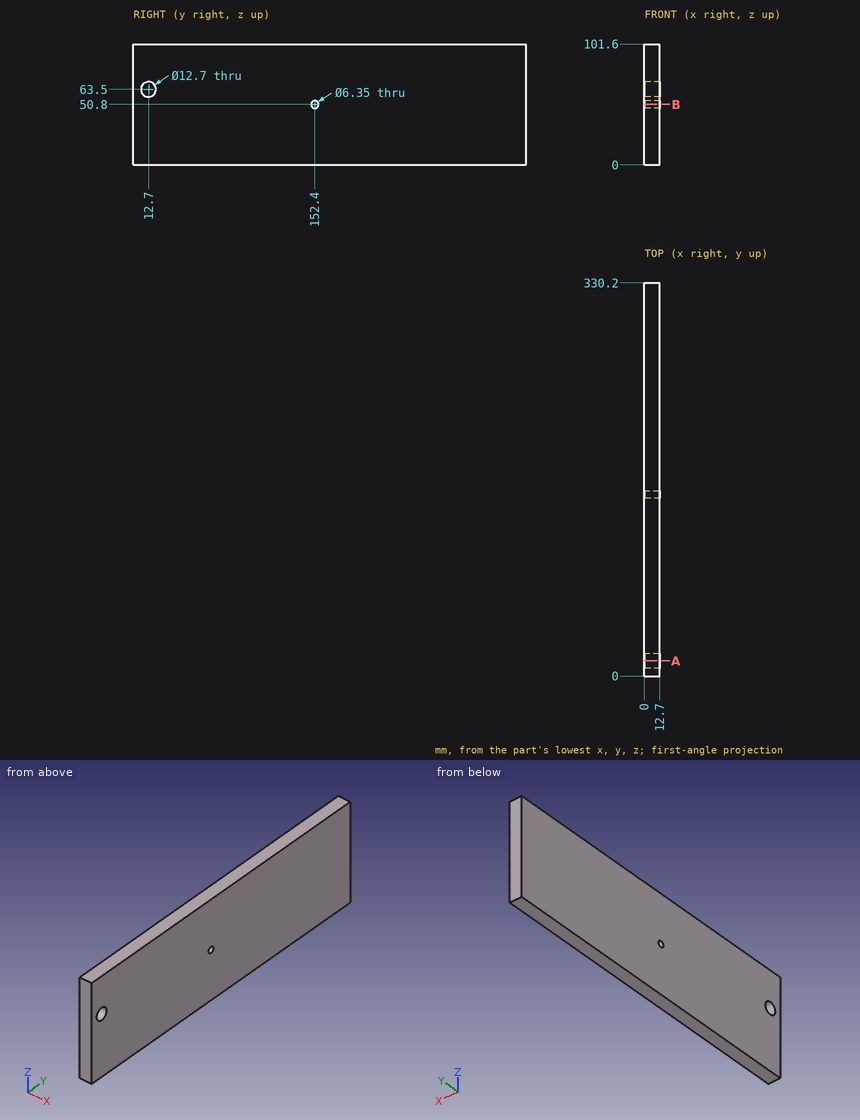
Drawing for the job (mm, zero at the part's lowest x, y, z). Give positions to 0.01 mm unless a question says otherwise; leave off trailing zeros. Order: outer loops, then holes, each group sorted by start corner. A loop starts at its lowest first (then second) coordinate and runs counter-clockwise, first axis right, second up. Notation, with made-up numbers: M -4.75,-6.75 L 13.25,-6.75 A31 ccw 13.25,28.25 Z; hole C 12.5,76 d7. An arc over 180 degrees is marked long. Put each result on its own line as item: value.
Item 1: Probe line 1 (Z direction, x = 3.25, y = 12.7); line 2 (Z direction, x = 9, y = 14). List the from-to ranges inside material, lowest first. Write a range as [from, to].
From the geometry:
line 1: z = [0, 57.15], [69.85, 101.6]
line 2: z = [0, 57.28], [69.72, 101.6]
Item 2: Flat gauge pin, fed straight in: pin 1 Ø5.5 at (y, z) = (152.4, 50.8) entering from -X. Where does the tip first touch, or does it go through?
From the geometry:
pin 1: passes through
Item 3: Slice it at A-A, the plane y = 12.7. Write the cut outline in (x, z), plus the area to 3 significant figures.
From the geometry:
outline: M 0,0 L 12.7,0 L 12.7,57.15 L 0,57.15 Z; M 0,69.85 L 12.7,69.85 L 12.7,101.6 L 0,101.6 Z
area: 1,130 mm2
Item 4: Slice it at B-B, the plane z = 50.8. Write the cut outline in (x, y) (3 decimals), plus the area to 3 significant figures.
From the geometry:
outline: M 0,0 L 12.7,0 L 12.7,149.225 L 0,149.225 Z; M 0,155.575 L 12.7,155.575 L 12.7,330.2 L 0,330.2 Z
area: 4,110 mm2
